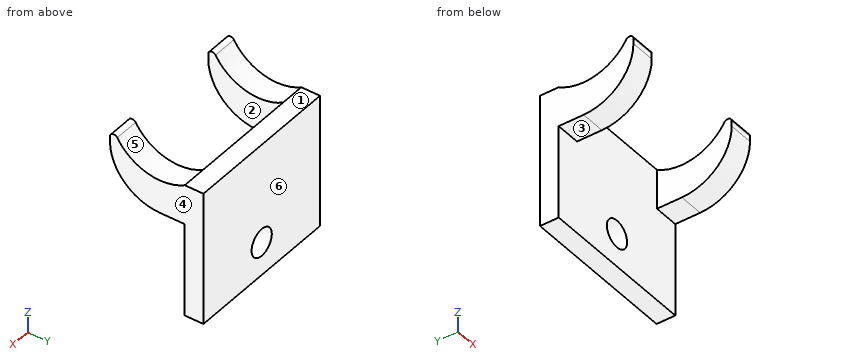
from build123d import *

# Parameters (mm, degrees)
SKETCH1_W            = 40.40124
SKETCH1_H            = 34.036
SKETCH1_R            = 1.257288094
BOSS_EXTRUDE1_DEPTH  = 4.7625
M6_CLEARANCE_HOLE1_D = 7
BOSS_EXTRUDE3_DEPTH  = 6.35
FILLET2_R            = 1
FILLET3_R            = 12.7


with BuildPart() as part:
    # Sketch1 → Boss-Extrude1 (new body)
    with BuildSketch(Plane(origin=(0, 0, 0), x_dir=(1, 0, 0), z_dir=(0, 1, 0))):
        with Locations((20.20062, 17.018)):
            Rectangle(SKETCH1_W, SKETCH1_H)
        with Locations(Location((20.20062, 25.522416525, 0), (0, 0, 90))):
            Circle(SKETCH1_R, mode=Mode.SUBTRACT)
    extrude(amount=BOSS_EXTRUDE1_DEPTH)

    # M6 Clearance Hole1 (through all)
    with Locations(Plane(origin=(0, 4.7625, 0), x_dir=(1, 0, 0), z_dir=(0, 1, 0))):
        with Locations((20.20062, 25.522416525)):
            Hole(M6_CLEARANCE_HOLE1_D / 2)

    # Sketch5 → Boss-Extrude3 (add)
    with BuildSketch(Plane(origin=(40.40124, 0, 0), x_dir=(0, 0, -1), z_dir=(1, 0, 0))):
        with BuildLine():
            Line((-10.998522628, -19.05), (10.16, -19.05))
            Line((10.16, -19.05), (10.16, 0))
            Line((10.16, 0), (0, 0))
            ThreePointArc((0, 0), (0, -12.7), (-10.998522628, -19.05))
        make_face()
    boss_extrude3 = extrude(amount=-BOSS_EXTRUDE3_DEPTH)

    # Mirror1: Boss-Extrude3 across plane
    add(boss_extrude3.mirror(Plane(origin=(20.20062, 0, 0), x_dir=(0, 0, 1), z_dir=(1, 0, 0))))

    # Fillet2
    fillet2_edges = [part.edges().sort_by_distance(p)[0] for p in [
        (37.22624, -19.05, 10.998522628),
        (3.175, -19.05, 10.998522628),
    ]]
    fillet(fillet2_edges, radius=FILLET2_R)

    # Fillet3
    fillet3_edges = [part.edges().sort_by_distance(p)[0] for p in [
        (37.22624, -19.05, -10.16),
        (3.175, -19.05, -10.16),
    ]]
    fillet(fillet3_edges, radius=FILLET3_R)


solid = part.part
Geometry: final body of the model. Coordinates: model frame, mm. Face numbers are marked on the shaded views. A direction names the side the tool comes from. Round coordinates to 2 decimals unless told otherwise and drop trailing zeros. Loops run counter-clockwise (first coordinate to the right, second up) from the corner with the lowest first, then second, coordinate; pieces in that order, holes last. Notation, with made-up numbers: (20, 77) - (33, 77) arc R23 cw to (33, 113) - close; hole circle Ø6 at (76.25, 9.5). An arc over 180 degrees is marked (long way). Write each question's results on one line, items separated by ' | '. Start each with the question number.
1) Line query: probe 1 along X at (y, z) = (-8, -3); probe 2 along Z at (x, y) = (28, 0.5); probe 3 along Y at (x, z) = (31, -16). Output: solid intervals per line, ascending. Write a range as [from, to].
2) First-contact query: P1, Ø2.5, axis at x = 15.5, y = 3, coming from the +Z side; P2, Ø7, axis at x = 2, y = -4, coming from the -Z side; P3, Ø1.5, axis at x = 9, z = -5.5, coming from the -Y side; P4, Ø5.5, axis at x = 20.2, z = -25.52, coming from the +Y side. Flat tips, straight axial feed; report the tip coordinate or a pass-through.
3) Cut plane A-A on z = -28.5. Return loops of the section in (x, y), then the cut area to 3 significant figures.
4) Access query for the marked faces 1, 2 and 3. Directions: +Z, -Z, +X, -X, +Y, -Y. A direction counts if a zero-diameter tool reaches every point of the face in a straight line with its end or side. Return the directions, or none.
5) Cut plane C-C on y = 2.5. Return loops of the section in (x, z), then the cut area to 3 significant figures.
6) Mould query, pull axis Y, two halves, no side actions, for the marked faces 4, 5 and 6. Classes: released by +Y, released by -Y, zero draft, split by the parting line, or undercut.
7) Cut plane D-D on z = -11. Return loops of the section in (x, y).
8) Cut plane B-B on x = 18. Return loops of the section in (y, z), then the cut area to 3 significant figures.
Verdict:
1) probe 1: x = [0, 6.35], [34.05, 40.4] | probe 2: z = [-34.04, 0] | probe 3: y = [0, 4.76]
2) P1: stops at z = 0 | P2: stops at z = -10.16 | P3: stops at y = 0 | P4: passes through
3) outline: (0, 0) - (18.36, 0) - (18.36, 4.76) - (0, 4.76) - close; (22.04, 0) - (40.4, 0) - (40.4, 4.76) - (22.04, 4.76) - close | area: 175 mm2
4) face 1: +Z, +X, -X, +Y | face 2: +Z, -Z, -Y | face 3: -Z, +X, -X, -Y
5) outline: (0, -34.04) - (40.4, -34.04) - (40.4, 0) - (0, 0) - close; hole circle Ø7 at (20.2, -25.52) | area: 1,340 mm2
6) face 4: zero draft | face 5: undercut | face 6: released by +Y
7) outline: (0, 0) - (40.4, 0) - (40.4, 4.76) - (0, 4.76) - close
8) outline: (0, -34.04) - (4.76, -34.04) - (4.76, -28.24) - (0, -28.24) - close; (0, -22.8) - (4.76, -22.8) - (4.76, 0) - (0, 0) - close | area: 136 mm2
